Verification items for the finished model (mm, model axes). Face numbers are marked on the shaded views. A direction names the side the tool comes from. Give positions to 0.01 mm unless a question says otherwise; leave off trailing zeros. Loops run counter-clockwise (first coordinate to the right, second up) from the corner with the lowest first, then second, coordinate; pieces in that order, holes last. Notation, with made-up numbers: (5.5, -38.5) - (51.5, -38.5) arc R27 ccw to (51.5, -6.5) - close; hole circle Ø6 at (-36.5, -30). An arc over 180 degrees is marked (long way). Answer in a Markdown table with one row per item.
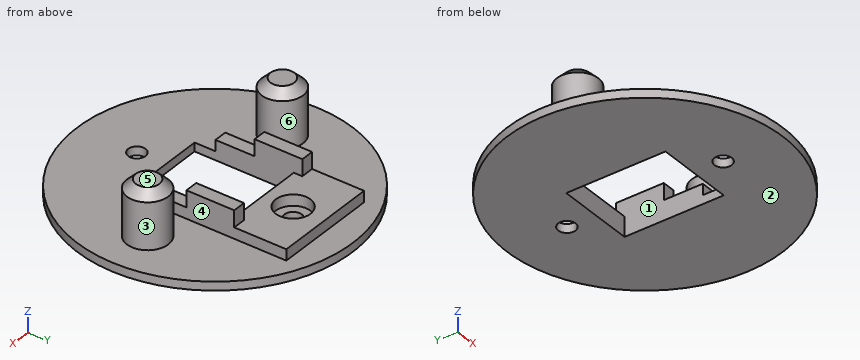
```python
from build123d import *

# Parameters (mm, degrees)
F0_R     = 15.875
F0_R_2   = 1
F0_W     = 9
F0_H     = 11.43
F1_DEPTH = 1
F2_R     = 2
F3_DEPTH = 1.27
F4_W     = 1.5
F4_H     = 5.5
F5_DEPTH = 1.905
F6_R     = 2.38125
F7_DEPTH = 6.35
F8_SIZE  = 1.016


# Not quite as in the source:
# - a pattern or mirror of a feature is missing from the dataset's text; its kind, count and spacing are read off the source's solid


with BuildPart() as f1:
    # F0 (on Top) → F1 (new body)
    with BuildSketch(Plane.XY):
        Circle(F0_R)
        with Locations((0, -9)):
            Circle(F0_R_2, mode=Mode.SUBTRACT)
        Rectangle(F0_W, F0_H, mode=Mode.SUBTRACT)
        with Locations((0, 9)):
            Circle(F0_R_2, mode=Mode.SUBTRACT)
    extrude(amount=F1_DEPTH)

    # F2 (on face) → F3 (join)
    with BuildSketch(Plane.XY.offset(1)):
        Polygon((6, 12.6974700204), (-6, 12.6974700204), (-6, -3.3025299796), (-4.5, -3.3025299796), (-4.5, 5.715), (4.5, 5.715), (4.5, -3.3025299796), (6, -3.3025299796), align=None)
        with Locations((0, 9)):
            Circle(F2_R, mode=Mode.SUBTRACT)
    extrude(amount=F3_DEPTH)

    # F4 (on face) → F5 (join)
    with BuildSketch(Plane.XY.offset(2.27)):
        with Locations((-5.25, 3.9474700204)):
            Rectangle(F4_W, F4_H)
    f5 = extrude(amount=F5_DEPTH)

    # F5_copies: F5 across plane
    add(f5.mirror(Plane(origin=(0, 0, 0), x_dir=(0, 0, 1), z_dir=(1, 0, 0))))

    # F6 (on face) → F7 (join)
    with BuildSketch(Plane.XY.offset(1)):
        with Locations((10.3898039088, 0)):
            Circle(F6_R)
        with Locations((-10.3898039088, 0)):
            Circle(F6_R)
    extrude(amount=F7_DEPTH)

    # F8
    f8_edges = [f1.edges().sort_by_distance(p)[0] for p in [
        (-12.771054, 0, 7.35),
        (8.008554, 0, 7.35),
    ]]
    chamfer(f8_edges, length=F8_SIZE)


solid = f1.part
```
Q1. Sectioned sample at C-C (y = 0). Record the cut outline in (x, z) (3 decimals).
Completed:
| item | result |
|---|---|
| outline | (-15.875, 0) - (-4.5, 0) - (-4.5, 2.27) - (-6, 2.27) - (-6, 1) - (-8.009, 1) - (-8.009, 6.334) - (-9.025, 7.35) - (-11.755, 7.35) - (-12.771, 6.334) - (-12.771, 1) - (-15.875, 1) - close; (4.5, 0) - (15.875, 0) - (15.875, 1) - (12.771, 1) - (12.771, 6.334) - (11.755, 7.35) - (9.025, 7.35) - (8.009, 6.334) - (8.009, 1) - (6, 1) - (6, 2.27) - (4.5, 2.27) - close |
Q2. Draft check along X on the marked faces 1, 2 and 3. Enter one of: +X half, -X half, draft (parallel to the pull), parting line (faces both ways), or undercut.
Completed:
| item | result |
|---|---|
| face 1 | undercut |
| face 2 | draft |
| face 3 | undercut |
Q3. Sectioned sample at B-B (z = 3). Record the cut outline in (x, y), and give its area (3 significant figures).
Completed:
| item | result |
|---|---|
| outline | circle Ø4.76 at (-10.39, 0); (-6, 1.2) - (-4.5, 1.2) - (-4.5, 6.7) - (-6, 6.7) - close; (4.5, 1.2) - (6, 1.2) - (6, 6.7) - (4.5, 6.7) - close; circle Ø4.76 at (10.39, 0) |
| area | 52.1 mm^2 |
Q4. Thickness scan on line 1 (Z direction, x = -5, y = 1); line 2 (Z direction, x = 7, y = 3); line 3 (X direction, y = 6, z = 3.75). Record the ranges inside material, lowest first.
Completed:
| item | result |
|---|---|
| line 1 | 0 to 2.27 |
| line 2 | 0 to 1 |
| line 3 | -6 to -4.5, 4.5 to 6 |
Q5. Tool access check on the marked faces 4, 5 and 6. Record the directions out of +Z, -Z, +X, -X, +Y, -Y that give a thin tool (end or side, any length) a straight path to the whole face; none if there is none.
Completed:
| item | result |
|---|---|
| face 4 | +Z, +Y, -Y |
| face 5 | +Z, +X, -X, +Y, -Y |
| face 6 | +Z |
Q6. Go/stop test with flat-tipped pins: P1, Ø1.2, axis at x = -0.5, y = 9, coming from the +Z side; P2, Ø8, axis at x = 3, y = 10, coming from the +Z side (3 decimals); P3, Ø0.6, axis at x = 5.5, z = 2, coming from the -Y side. Record where each tip stops, or that it passes through.
Completed:
| item | result |
|---|---|
| P1 | z = 1 |
| P2 | z = 4.175 |
| P3 | y = -3.3 |
Q7. Sectioned sample at D-D (y = 9). Record the cut outline in (x, z).
Completed:
| item | result |
|---|---|
| outline | (-13.08, 0) - (-1, 0) - (-1, 1) - (-2, 1) - (-2, 2.27) - (-6, 2.27) - (-6, 1) - (-13.08, 1) - close; (1, 0) - (13.08, 0) - (13.08, 1) - (6, 1) - (6, 2.27) - (2, 2.27) - (2, 1) - (1, 1) - close |
Q8. Sectioned sample at A-A (x = 0). Record the cut outline in (y, z) (3 decimals), and give its area (3 significant figures).
Completed:
| item | result |
|---|---|
| outline | (-15.875, 0) - (-10, 0) - (-10, 1) - (-15.875, 1) - close; (-8, 0) - (-5.715, 0) - (-5.715, 1) - (-8, 1) - close; (5.715, 0) - (8, 0) - (8, 1) - (7, 1) - (7, 2.27) - (5.715, 2.27) - close; (10, 0) - (15.875, 0) - (15.875, 1) - (12.697, 1) - (12.697, 2.27) - (11, 2.27) - (11, 1) - (10, 1) - close |
| area | 20.1 mm^2 |
